The model under review builds one solid part; all positions refer to its coordinate system, in mm. Face numbers are marked on the shaded views. A direction names the side the tool comes from. Coordinates: 2 decimals unless noted, no trailing zeros. Order: outer loops, then holes, each group sorted by start corner. A loop starts at its lowest first (then second) coordinate and runs counter-clockwise, first axis right, second up. Notation, with made-up numbers: (10, -1) -> (24, -1) arc R15 cw to (24, 7) -> close; hole circle Ø8 at (55.25, 32). An arc over 180 degrees is marked (long way). Use one line per item in the form item = value. Start each with the question number.
(1) Insertion check: pin 1 Ø6 at (y, z) = (11, 5) entering from +X; pin 2 Ø2 at (x, z) = (-11, 0) entering from -Y; pin 3 Ø1.5 at (x, z) = (0.5, -9.5) entering from +Y; pin 4 Ø1 at (x, z) = (1, 6) entering from +Y. Each pin has a flat end and moves straight along its axis. Give the tip position at first contact, or say it passes through.
(2) Wall thickness on line 1 along Z through (x, y) = (0, 4.25); line 2 along Z through (x, y) = (0, 1.3); line 3 along Z through (x, y) = (6.75, -2): over which ranges is each line inside the solid? List them lowest first.
(3) Mouldability with a two-part tool opening along Z and no side actions: class the marked faces 4, 5 and 6 as +Z half, -Z half, draft (parallel to the pull), parting line (faces both ways), or undercut.
(4) Take a section at B-B (z = 11). State the section outline as (x, y) points, then the cut area to 3 significant figures.
(5) For the marked faces 1, 2 and 3, list the 3-axis set-ups (+Z, -Z, +X, -X, +Y, -Y) from which the entire face can be reached by the end or side of a thin tool; tool diameter is ignored.
(6) Take a section at A-A (x = 0). State the section outline as (y, z) points, then the cut area to 3 significant figures.
(7) Take a section at D-D (x = -11). State the section outline as (y, z) points, then the cut area to 3 significant figures.
(8) Take a section at C-C (y = -1). State how many separate pieces and enclosed holes the cut face has, then the cut area to 3 significant figures.
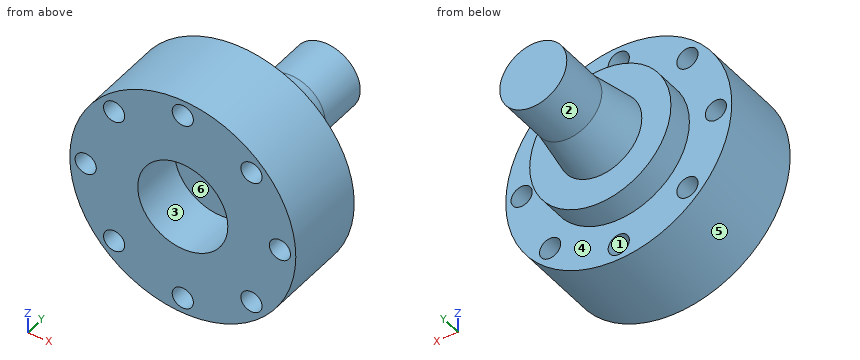
```python
from build123d import *

# Parameters (mm, degrees)
SKETCH_1_R           = 12.8
EXTRUDE_1_DEPTH      = 9.5
EXTRUDE_1_DEPTH_BACK = 3
SKETCH_24_R          = 1.2
CUT_EXTRUDE_1_DEPTH  = 24.4
SKETCH_25_R          = 5.1
CUT_EXTRUDE_2_DEPTH  = 6
SKETCH_26_R          = 12.8
SKETCH_26_R_2        = 8
CUT_EXTRUDE_4_DEPTH  = 3


with BuildPart() as part:
    # 스케치1 → 보스-돌출1 (new body, two sides)
    with BuildSketch(Plane(origin=(0, 0, 0), x_dir=(1, 0, 0), z_dir=(0, 1, 0))) as extrude_1_sk:
        Circle(SKETCH_1_R)
    extrude(amount=EXTRUDE_1_DEPTH)
    extrude(extrude_1_sk.sketch, amount=-EXTRUDE_1_DEPTH_BACK)

    # 스케치18 → 회전1 (revolve)
    with BuildSketch(Plane.XY):
        Polygon((0, 9.5), (-4.7, 9.5), (-3.8, 14.7), (-3.8, 20.4), (0, 20.4), (0, 14.7), align=None)
    revolve(axis=Axis((0, 15.188164867, 0), (0, -1, 0)))

    # 스케치24 → 컷-돌출1 (cut, through all)
    with BuildSketch(Plane.XZ.offset(3)):
        with Locations((0, 11)):
            Circle(SKETCH_24_R)
        with Locations((7.778174593, 7.778174593)):
            Circle(SKETCH_24_R)
        with Locations((11, 0)):
            Circle(SKETCH_24_R)
        with Locations((0, -11)):
            Circle(SKETCH_24_R)
        with Locations((-7.778174593, -7.778174593)):
            Circle(SKETCH_24_R)
        with Locations((-7.778174593, 7.778174593)):
            Circle(SKETCH_24_R)
        with Locations((7.778174593, -7.778174593)):
            Circle(SKETCH_24_R)
        with Locations((-11, 0)):
            Circle(SKETCH_24_R)
    extrude(amount=-CUT_EXTRUDE_1_DEPTH, mode=Mode.SUBTRACT)

    # 스케치25 → 컷-돌출2 (cut)
    with BuildSketch(Plane.XZ.offset(3)):
        Circle(SKETCH_25_R)
    extrude(amount=-CUT_EXTRUDE_2_DEPTH, mode=Mode.SUBTRACT)

    # 스케치26 → 컷-돌출4 (cut)
    with BuildSketch(Plane(origin=(0, 9.5, 0), x_dir=(1, 0, 0), z_dir=(0, 1, 0))):
        Circle(SKETCH_26_R)
        Circle(SKETCH_26_R_2, mode=Mode.SUBTRACT)
    extrude(amount=-CUT_EXTRUDE_4_DEPTH, mode=Mode.SUBTRACT)


solid = part.part
```
Findings:
q1.pin_1 = 7.63
q1.pin_2 = through
q1.pin_3 = 6.5
q1.pin_4 = 9.5
q2.line_1 = -12.8 to -12.2, -9.8 to 9.8, 12.2 to 12.8
q2.line_2 = -12.8 to -12.2, -9.8 to -5.1, 5.1 to 9.8, 12.2 to 12.8
q2.line_3 = -10.88 to -8.4, -7.16 to 7.16, 8.4 to 10.88
q3.face_4 = draft
q3.face_5 = parting line
q3.face_6 = undercut
q4.outline = (-6.55, -3) -> (-1.2, -3) -> (-1.2, 6.5) -> (-6.55, 6.5) -> close; (1.2, -3) -> (6.55, -3) -> (6.55, 6.5) -> (1.2, 6.5) -> close
q4.area = 102 mm²
q5.face_1 = +Y, -Y
q5.face_2 = +Y
q5.face_3 = -Y
q6.outline = (-3, -12.8) -> (6.5, -12.8) -> (6.5, -12.2) -> (-3, -12.2) -> close; (-3, -9.8) -> (6.5, -9.8) -> (6.5, -8) -> (9.5, -8) -> (9.5, -4.7) -> (14.7, -3.8) -> (20.4, -3.8) -> (20.4, 3.8) -> (14.7, 3.8) -> (9.5, 4.7) -> (9.5, 8) -> (6.5, 8) -> (6.5, 9.8) -> (-3, 9.8) -> (-3, 5.1) -> (3, 5.1) -> (3, -5.1) -> (-3, -5.1) -> close; (-3, 12.2) -> (6.5, 12.2) -> (6.5, 12.8) -> (-3, 12.8) -> close
q6.area = 272 mm²
q7.outline = (-3, -6.55) -> (6.5, -6.55) -> (6.5, -1.2) -> (-3, -1.2) -> close; (-3, 1.2) -> (6.5, 1.2) -> (6.5, 6.55) -> (-3, 6.55) -> close
q7.area = 102 mm²
q8.separate_pieces = 1
q8.enclosed_holes = 9
q8.area = 397 mm²
